Here's how the part is built. I have some questions about the finished solid (model axes, mm). A direction names the side the tool comes from. Round coordinates to 2 decimals unless told otherwise and drop trailing zeros. Write each loop counter-clockwise with the first axis right and the second up, starting at its lowest first coordinate (ties: lowest second). Pieces come first, ordered by that corner, then holes. Notation, with made-up numbers: (-14, 80.5) - (27, 80.5) arc R20 cw to (27, 92.5) - close; hole circle Ø8 at (13, 50.25). An arc over 180 degrees is marked (long way). One line per question, with ' | ' between items. Start each with the question number.
(1) Imagine slicing it at B-B (x = -17). Write out the boundary of the cut face in (y, z), plus the area to 3 significant figures.
(2) Imagine slicing it at C-C (y = 15.5). Write out the boundary of the cut face in (x, z).
(3) Thinking about a two-plate mould opening in X: for faces 3 (the flat face through (0, 0, 12.7)), 4 (the flat face through (17.666, 10, 0)), 5 (the cylindrical face through (18.4, -9, 0.2)), 6 (the flat face through (-20.638, 0, 0)), which applies, pulls with the +X half, pulls with the -X half, needs draft (parallel to the pull), parting line crosses it, or undercut?
(4) Imagine slicing it at A-A (y = -10). Write out the boundary of the cut face in (x, z).
(5) For faces 1 (the flat face through (17.666, -10, 0)), 2 (the flat face through (11.112, 20, 0)), which set-ups out of +Z, -Z, +X, -X, +Y, -Y let a thin tool reach every point of the face, with its end or its side?
(6) Imagine slicing it at D-D (x = -3). Write out the boundary of the cut face in (y, z), plus the area to 3 significant figures.
(7) Will these pins go through, and if not, where does the flat tip stop? pin 1 (7.5 mm diameter, centred on x = -0.5, z = 4.5, fed in from -Y); pin 2 (7.5 mm diameter, centred on x = 0.5, z = -5.5, fed in from +Y).
(8) If I drill on L1, parallel to Y at x = 15, z = -6.5; L2, parallel to X at y = 16.5, z = 4.25; L3, parallel to X at y = -11, z = -9.5, over which ranges is the centre line in solid material (lowest first)?
from build123d import *

# Parameters (mm, degrees)
BASE_EXTRUDE_DEPTH = 12.7
FILLET1_R          = 0.9906


with BuildPart() as part:
    # Sketch1 → Base-Extrude (new, symmetric)
    with BuildSketch(Plane.XY):
        with BuildLine():
            Line((-11.1125, 20.6375), (-20.6375, 20.6375))
            Line((-20.6375, 20.6375), (-20.6375, -20.6375))
            Line((-20.6375, -20.6375), (-11.1125, -20.6375))
            Line((-11.1125, -20.6375), (-11.1125, -18.6563))
            Line((-11.1125, -18.6563), (-12.256346355, -16.6751))
            Line((-12.256346355, -16.6751), (-13.400192707, -18.6563))
            Line((-13.400192707, -18.6563), (-17.6657, -18.6563))
            ThreePointArc((-17.6657, -18.6563), (-18.366159977, -18.366159977), (-18.6563, -17.6657))
            Line((-18.6563, -17.6657), (-18.6563, -11.30935))
            Line((-18.6563, -11.30935), (-17.6657, -11.30935))
            Line((-17.6657, -11.30935), (-17.6657, -9.32815))
            Line((-17.6657, -9.32815), (-18.6563, -9.32815))
            Line((-18.6563, -9.32815), (-18.6563, -1.9812))
            ThreePointArc((-18.6563, -1.9812), (-18.366159977, -1.280740023), (-17.6657, -0.9906))
            Line((-17.6657, -0.9906), (17.6657, -0.9906))
            ThreePointArc((17.6657, -0.9906), (18.366159977, -1.280740023), (18.6563, -1.9812))
            Line((18.6563, -1.9812), (18.6563, -9.32815))
            Line((18.6563, -9.32815), (17.6657, -9.32815))
            Line((17.6657, -9.32815), (17.6657, -11.30935))
            Line((17.6657, -11.30935), (18.6563, -11.30935))
            Line((18.6563, -11.30935), (18.6563, -17.6657))
            ThreePointArc((18.6563, -17.6657), (18.366159977, -18.366159977), (17.6657, -18.6563))
            Line((17.6657, -18.6563), (13.400192707, -18.6563))
            Line((13.400192707, -18.6563), (12.256346355, -16.6751))
            Line((12.256346355, -16.6751), (11.1125, -18.6563))
            Line((11.1125, -18.6563), (11.1125, -20.6375))
            Line((11.1125, -20.6375), (20.6375, -20.6375))
            Line((20.6375, -20.6375), (20.6375, 20.6375))
            Line((20.6375, 20.6375), (11.1125, 20.6375))
            Line((11.1125, 20.6375), (11.1125, 18.6563))
            Line((11.1125, 18.6563), (12.256346355, 16.6751))
            Line((12.256346355, 16.6751), (13.400192707, 18.6563))
            Line((13.400192707, 18.6563), (17.6657, 18.6563))
            ThreePointArc((17.6657, 18.6563), (18.366159977, 18.366159977), (18.6563, 17.6657))
            Line((18.6563, 17.6657), (18.6563, 11.30935))
            Line((18.6563, 11.30935), (17.6657, 11.30935))
            Line((17.6657, 11.30935), (17.6657, 9.32815))
            Line((17.6657, 9.32815), (18.6563, 9.32815))
            Line((18.6563, 9.32815), (18.6563, 1.9812))
            ThreePointArc((18.6563, 1.9812), (18.366159977, 1.280740023), (17.6657, 0.9906))
            Line((17.6657, 0.9906), (-17.6657, 0.9906))
            ThreePointArc((-17.6657, 0.9906), (-18.366159977, 1.280740023), (-18.6563, 1.9812))
            Line((-18.6563, 1.9812), (-18.6563, 9.32815))
            Line((-18.6563, 9.32815), (-17.6657, 9.32815))
            Line((-17.6657, 9.32815), (-17.6657, 11.30935))
            Line((-17.6657, 11.30935), (-18.6563, 11.30935))
            Line((-18.6563, 11.30935), (-18.6563, 17.6657))
            ThreePointArc((-18.6563, 17.6657), (-18.366159977, 18.366159977), (-17.6657, 18.6563))
            Line((-17.6657, 18.6563), (-13.400192707, 18.6563))
            Line((-13.400192707, 18.6563), (-12.256346355, 16.6751))
            Line((-12.256346355, 16.6751), (-11.1125, 18.6563))
            Line((-11.1125, 18.6563), (-11.1125, 20.6375))
        make_face()
    extrude(amount=BASE_EXTRUDE_DEPTH, both=True)

    # Fillet1
    fillet1_edges = [part.edges().sort_by_distance(p)[0] for p in [
        (18.6563, 11.30935, 0),
        (18.6563, -9.32815, 0),
        (-18.6563, 11.30935, 0),
        (-18.6563, -9.32815, 0),
        (-18.6563, 9.32815, 0),
        (-18.6563, -11.30935, 0),
        (18.6563, 9.32815, 0),
        (18.6563, -11.30935, 0),
    ]]
    fillet(fillet1_edges, radius=FILLET1_R - 0.0001)  # a hair under: the kernel refuses the full size


solid = part.part
Check sheet entries:
1) outline: (-20.64, -12.7) - (-18.66, -12.7) - (-18.66, 12.7) - (-20.64, 12.7) - close; (-0.99, -12.7) - (0.99, -12.7) - (0.99, 12.7) - (-0.99, 12.7) - close; (18.66, -12.7) - (20.64, -12.7) - (20.64, 12.7) - (18.66, 12.7) - close | area: 151 mm^2
2) outline: (-20.64, -12.7) - (-18.66, -12.7) - (-18.66, 12.7) - (-20.64, 12.7) - close; (18.66, -12.7) - (20.64, -12.7) - (20.64, 12.7) - (18.66, 12.7) - close
3) face 3: needs draft | face 4: undercut | face 5: undercut | face 6: pulls with the -X half
4) outline: (-20.64, -12.7) - (-17.67, -12.7) - (-17.67, 12.7) - (-20.64, 12.7) - close; (17.67, -12.7) - (20.64, -12.7) - (20.64, 12.7) - (17.67, 12.7) - close
5) face 1: +Z, -Z | face 2: +Z, -Z, +Y
6) outline: (-0.99, -12.7) - (0.99, -12.7) - (0.99, 12.7) - (-0.99, 12.7) - close | area: 50.3 mm^2
7) pin 1: y = -0.99 | pin 2: y = 0.99
8) L1: -20.64 to -18.66, -0.99 to 0.99, 18.66 to 20.64 | L2: -20.64 to -18.66, 18.66 to 20.64 | L3: -20.64 to -17.67, 17.67 to 20.64
